from build123d import *

# Parameters (mm, degrees)
SKETCH3_W = 14
SKETCH3_H = 6


with BuildPart() as part:
    # Sweep1: sweep along a path in Sketch2
    with BuildLine(Plane.XY) as sweep1_path:
        Line((64.14139557, 7.274636075), (66.044393052, 31.114017371))
        ThreePointArc((66.044393052, 31.114017371), (75.895604213, 43.384839753), (90.932163332, 38.745730666))
        Line((90.932163332, 38.745730666), (210.932163332, -111.254269334))
        ThreePointArc((210.932163332, -111.254269334), (212.618245308, -126.064642227), (200, -134))
        Line((200, -134), (-50, -134))
        ThreePointArc((-50, -134), (-59.899494937, -129.899494937), (-64, -120))
        Line((-64, -120), (-64, 27.282396409))
        ThreePointArc((-64, 27.282396409), (-54.981361234, 40.366204733), (-39.544851392, 36.593135778))
        Line((-39.544851392, 36.593135778), (4.422225727, -12.778058812))
        ThreePointArc((4.422225727, -12.778058812), (40.902364216, -22.46846092), (64.14139557, 7.274636075))
    # Sketch3 → Sweep1 (sweep)
    with BuildSketch(Plane(origin=(-50, -134, 0), x_dir=(0, 0, 1), z_dir=(-1, 0, 0))):
        Rectangle(SKETCH3_W, SKETCH3_H)
    sweep(path=sweep1_path.line)


solid = part.part
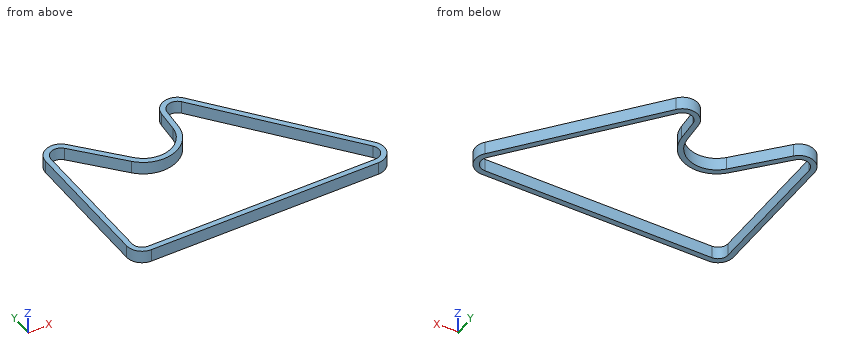
For this review, take the finished solid that the model builds, in its own axes (mm). Give positions to 0.01 mm unless a question says otherwise; leave off trailing zeros. Order: outer loops, then holes, each group sorted by start corner. A loop starts at its lowest first (then second) coordinate and runs counter-clockwise, first axis right, second up. Notation, with made-up numbers: (39.5, 3.25) - (77.5, 3.25) arc R17 cw to (77.5, 17.25) - close; hole circle Ø6 at (-9.5, -18.75). An arc over 180 degrees is marked (long way). Answer as a JSON object with one key per item and string values. Group by question number.
Item 1: Wall thickness on line 1 along X through (y, z) = (27, 1); line 2 along X through (y, z) = (-0.5, -1.25); line 3 along Y through (x, z) = (28, 1.75): over which ranges is each line inside the solid? List them lowest first.
Item 2: Take a section at C-C on x = 20. Give the boundary of the cut face in (y, z), and give its area (3 significant figures).
Item 3: Clearance check with flat-ended pins moving along their axes: pin 1 Ø4 at (y, z) = (-73.5, -1.5) entering from +X; pin 2 Ø4 at (x, z) = (-27.5, 0.5) entering from +Y; pin 3 Ø3 at (x, z) = (88, -3.5) entering from +Y; pin 4 Ø6 at (x, y) = (170.5, -66) entering from -Z. State where each tip first meets the part, or that it passes through.
Item 4: Take a section at D-D on y = -106. Give the boundary of the cut face in (x, z).
Item 5: Take a section at B-B on y = 11.5. Give the boundary of the cut face in (x, z).
Item 6: Take a section at A-A on z = -4. Give the boundary of the cut face in (x, y), and give its area (3 significant figures).
Reported:
{
 "1": {"line 1": "-67 to -61, -35.02 to -26.98, 62.71 to 68.73, 96.49 to 104.17", "line 2": "-67 to -61, -10.53 to -2.49, 59.43 to 65.74, 118.49 to 126.17", "line 3": "-137 to -131, -27.2 to -21.19"},
 "2": {"outline": "(-137, -7) - (-131, -7) - (-131, 7) - (-137, 7) - close; (-25.88, -7) - (-19.61, -7) - (-19.61, 7) - (-25.88, 7) - close", "area": "172 mm^2"},
 "3": {"pin 1": "x = 186.17", "pin 2": "y = 29.82", "pin 3": "y = 45.71", "pin 4": "z = -7"},
 "4": {"outline": "(-67, -7) - (-61, -7) - (-61, 7) - (-67, 7) - close; (202.89, -7) - (210.57, -7) - (210.57, 7) - (202.89, 7) - close"},
 "5": {"outline": "(-67, -7) - (-61, -7) - (-61, 7) - (-67, 7) - close; (-21.22, -7) - (-13.18, -7) - (-13.18, 7) - (-21.22, 7) - close; (61.47, -7) - (67.49, -7) - (67.49, 7) - (61.47, 7) - close; (108.89, -7) - (116.57, -7) - (116.57, 7) - (108.89, 7) - close"},
 "6": {"outline": "(-67, -120) arc R17 ccw to (-50, -137) - (200, -137) arc R17 ccw to (213.27, -109.38) - (93.27, 40.62) arc R17 ccw to (63.05, 31.35) - (61.15, 7.51) arc R31.25 cw to (6.66, -10.78) - (-37.3, 38.59) arc R17 ccw to (-67, 27.28) - close; hole (-61, -120) arc R11 ccw to (-50, -131) - (200, -131) arc R11 ccw to (208.59, -113.13) - (88.59, 36.87) arc R11 ccw to (69.03, 30.88) - (67.13, 7.04) arc R37.25 cw to (2.18, -14.77) - (-41.79, 34.6) arc R11 ccw to (-61, 27.28) - close", "area": "5,280 mm^2"}
}
